Source: CAD feature listing. Evaluate the final solid. Frame: model axes, mm. A direction names the side the tool comes from. Give positions to 0.01 mm unless a question says otherwise; leave off trailing zeros. Order: outer loops, then holes, each group sorted by start corner. A loop starts at its lowest first (then second) coordinate and runs counter-clockwise, first axis right, second up. Notation, with made-up numbers: (19.25, 52.25) - (43.25, 52.25) arc R26 ccw to (43.25, 86.25) - close; hole circle Ø11 at (12, 69). An arc over 180 degrees is marked (long way). Answer as CSV lines item,"result".
```python
from build123d import *

# Parameters (mm, degrees)
BOSS_EXTRUDE1_DEPTH = 3
SKETCH2_R           = 2
BOSS_EXTRUDE2_DEPTH = 18


with BuildPart() as part:
    # Sketch1 → Boss-Extrude1 (new body)
    with BuildSketch(Plane.XY):
        Polygon((3.33681456, -3.019216553), (4.283125514, 1.3801579), (0.946310955, 4.399374453), (-3.33681456, 3.019216553), (-4.283125514, -1.3801579), (-0.946310955, -4.399374453), align=None)
    extrude(amount=BOSS_EXTRUDE1_DEPTH)

    # Sketch2 → Boss-Extrude2 (add)
    with BuildSketch(Plane.XY.offset(3)):
        Circle(SKETCH2_R)
    extrude(amount=BOSS_EXTRUDE2_DEPTH)


solid = part.part
```
(1) Cut plane B-B (x = -0.75). Return loops of the section in (y, z).
Completed:
outline,"(-4.34, 0) - (3.85, 0) - (3.85, 3) - (1.85, 3) - (1.85, 21) - (-1.85, 21) - (-1.85, 3) - (-4.34, 3) - close"
(2) Cut plane D-D (x = 2.25). Return loops of the section in (y, z), then the cut area to 3 significant figures.
Completed:
outline,"(-3.37, 0) - (3.22, 0) - (3.22, 3) - (-3.37, 3) - close"
area,"19.8 mm²"
(3) Ray query, line 1 (Z direction, x = 2.25, y = -1.5); line 2 (Y direction, x = 0, z = 16.5); line 3 (X direction, y = -0.5, z = 19.75). Return the intervals inside material, ascending. Write a range as from..to.
Completed:
line 1,"0..3"
line 2,"-2..2"
line 3,"-1.94..1.94"
(4) Contact query for flat-ended pins moving along their axis: pin 1 (4 mm diameter, centred on x = 1.5, z = 13.5, fed in from -Y); pin 2 (2 mm diameter, centred on y = 2.5, z = 4.5, fed in from -X); pin 3 (2 mm diameter, centred on y = 0, z = 15.5, fed in from -X). Output: stop coordinate, or through.
Completed:
pin 1,"y = -2"
pin 2,"x = -1.32"
pin 3,"x = -2"
(5) Cut plane C-C (y = -1.75). Return loops of the section in (x, z), then the cut area to 3 significant figures.
Completed:
outline,"(-3.87, 0) - (3.61, 0) - (3.61, 3) - (0.97, 3) - (0.97, 21) - (-0.97, 21) - (-0.97, 3) - (-3.87, 3) - close"
area,"57.3 mm²"
(6) Access query for faces 1 (the flat face through (3.803, -0.85, 1.479)), 2 (the cylindrical face through (0, -2, 12)). Directions: +Z, -Z, +X, -X, +Y, -Y. A direction counts if a zero-diameter tool reaches every point of the face in a straight line with its end or side. Return the directions, or none.
Completed:
face 1,"+Z, -Z, +X, -Y"
face 2,"+Z"
(7) Cut plane A-A (z = 5.5). Return loops of the section in (x, y).
Completed:
outline,"circle Ø4 at (0, 0)"
